The listing builds one solid part. Answer for the finished solid, in the listing's coordinates (mm). Face numbers are marked on the shaded views. A direction names the side the tool comes from. Coordinates: 2 decimals unless noted, no trailing zeros. Write each loop counter-clockwise with the first axis right and the second up, starting at its lowest first coordinate (ties: lowest second). Pieces come first, ordered by that corner, then holes.
(1) The part is cut by section B-B on y = -0.75. Determine the outline of the cut face in (x, z), plus the area to 3 significant figures.
(2) Straight lines are drawn through the part: line 1 (Y direction, x = 12.5, z = 1.2); line 2 (Y direction, x = 6.75, z = 47.5); line 3 (Z direction, x = 3.75, y = 17). For each, find the intervals that lie inside material, in ascending order.
(3) The part is cut by section D-D on y = 11.5. Determine the outline of the cut face in (x, z).
(4) Which of the six approach directions +Z, -Z, +X, -X, +Y, -Y give full straight-line access (tool end or side, diameter ignored) to the marked faces 1 and 2?
(5) The part is cut by section A-A on x = 12.5. Determine the outline of the cut face in (y, z).
(6) Given P1, Ø6.5, axis at x = -7.5, y = 9.76, coming from the +Z side; P2, Ø9, axis at x = 3.5, z = 16.5, coming from the +Y side, each flat-ended and moving along its own axis, determine where each tip first touches the part or whether it passes through.
(7) The part is cut by section C-C on x = 3.25. Determine the outline of the cut face in (y, z), plus the area to 4 significant figures.
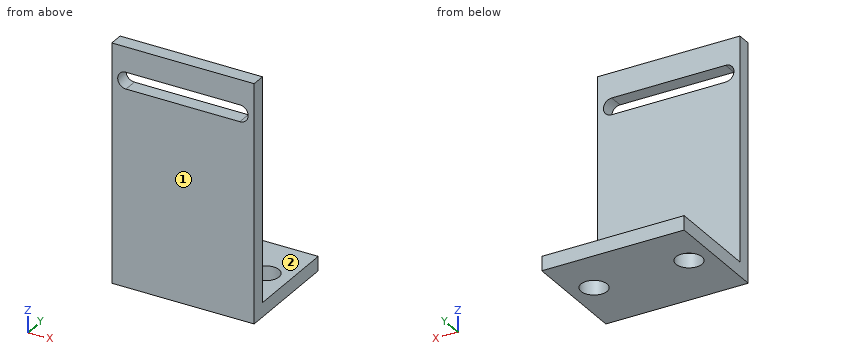
from build123d import *

# Parameters (mm, degrees)
F0_W     = 30
F0_H     = 50
F1_DEPTH = 3
F2_W     = 30
F2_H     = 3
F3_DEPTH = 20
F4_R     = 2.75
F5_DEPTH = 3.001
F7_DEPTH = 23.001


with BuildPart() as f1:
    # F0 (on Front) → F1 (new body)
    with BuildSketch(Plane.XZ):
        with Locations((2.5, 25)):
            Rectangle(F0_W, F0_H)
    extrude(amount=F1_DEPTH)

    # F2 (on face) → F3 (join)
    with BuildSketch(Plane(origin=(0, 0, 0), x_dir=(-1, 0, 0), z_dir=(0, 1, 0))):
        with Locations((-2.5, 1.5)):
            Rectangle(F2_W, F2_H)
    extrude(amount=F3_DEPTH)

    # F4 (on face) → F5 (cut, through all)
    with BuildSketch(Plane.XY.offset(3)):
        with Locations((12.5, 9.75894)):
            Circle(F4_R)
        with Locations((-7.5, 9.75894)):
            Circle(F4_R)
    extrude(amount=-F5_DEPTH, mode=Mode.SUBTRACT)

    # F6 (on face) → F7 (cut, through all)
    with BuildSketch(Plane.XZ.offset(3)):
        with BuildLine():
            Line((14.5, 44.75), (-9.5, 44.75))
            ThreePointArc((-9.5, 44.75), (-11.25, 43), (-9.5, 41.25))
            Line((-9.5, 41.25), (14.5, 41.25))
            ThreePointArc((14.5, 41.25), (16.25, 43), (14.5, 44.75))
        make_face()
    extrude(amount=-F7_DEPTH, mode=Mode.SUBTRACT)


solid = f1.part
Model answer:
1. outline: (-12.5, 0) - (17.5, 0) - (17.5, 50) - (-12.5, 50) - close; hole (-9.5, 41.25) - (14.5, 41.25) arc R1.75 ccw to (14.5, 44.75) - (-9.5, 44.75) arc R1.75 ccw to start
1. area: 1,410 mm2
2. line 1: y = -3 to 7.01, 12.51 to 20
2. line 2: y = -3 to 0
2. line 3: z = 0 to 3
3. outline: (-12.5, 0) - (-9.63, 0) - (-9.63, 3) - (-12.5, 3) - close; (-5.37, 0) - (10.37, 0) - (10.37, 3) - (-5.37, 3) - close; (14.63, 0) - (17.5, 0) - (17.5, 3) - (14.63, 3) - close
4. face 1: +Z, -Z, +X, -X, -Y
4. face 2: +Z, +X, -X, +Y
5. outline: (-3, 0) - (7.01, 0) - (7.01, 3) - (0, 3) - (0, 41.25) - (-3, 41.25) - close; (-3, 44.75) - (0, 44.75) - (0, 50) - (-3, 50) - close; (12.51, 0) - (20, 0) - (20, 3) - (12.51, 3) - close
6. P1: stops at z = 3
6. P2: stops at y = 0
7. outline: (-3, 0) - (20, 0) - (20, 3) - (0, 3) - (0, 41.25) - (-3, 41.25) - close; (-3, 44.75) - (0, 44.75) - (0, 50) - (-3, 50) - close
7. area: 199.5 mm2
